Autodesk Fusion 360 part; units mm, degrees
sketch "Sketch1" plane through (0, 0, 0) normal (0, 0, 1) x (1, 0, 0)
  line L0 (30, -70) -> (-30, -70)
  line L1 (-30, -70) -> (-30, 70)
  line L2 (-30, 70) -> (30, 70)
  line L3 (30, 70) -> (30, -70)
  line L4 (30, -70) -> (-30, 70) construction
  line L5 (-30, -70) -> (30, 70) construction
  line L6 (-30, 70) -> (10, 70)
  line L7 (10, 70) -> (10, 55)
  line L8 (10, 55) -> (-30, 55)
  line L9 (-30, 55) -> (-30, 70)
  line L10 (-30, 50) -> (-25, 50)
  line L11 (-25, 50) -> (-25, 34)
  line L12 (-25, 34) -> (-30, 34)
  line L13 (-30, 34) -> (-30, 50)
  line L14 (0, 1.75) -> (0, 22.5)
  line L15 (30, 50) -> (25, 50)
  line L16 (25, 50) -> (25, 34)
  line L17 (25, 34) -> (30, 34)
  line L18 (-30, 34) -> (-25, 34)
  line L19 (-25, 34) -> (-25, 24)
  line L20 (-25, 24) -> (-30, 24)
  line L21 (-30, 24) -> (-30, 34)
  line L22 (25, 34) -> (25, 24)
  line L23 (25, 24) -> (30, 24)
  line L24 (25, 34) -> (30, 34)
  dimension "d1" = 60
  dimension "d2" = 140
  dimension "d3" = 40
  dimension "d4" = 15
  dimension "d5" = 5
  dimension "d6" = 16
  dimension "d7" = 5
  dimension "d8" = 5
  dimension "d9" = 10
extrude "Extrude1" add sketch "Sketch1" along normal blind 4 contours L0 L1 L2 L3 L7 L8 L10 L11 L15 L16 L19 L20 L22 L23
extrude "Extrude2" add sketch "Sketch1" along normal blind 12 contours L3 L17 L22 L23 L24 | L1 L12 L18 L19 L20 L21
chamfer "Chamfer1" distance 15 distance2 30 1 edges at (30, -70, 2) measured on face at (10, -70, 1.3333)
chamfer "Chamfer1" distance 30 distance2 15 1 edges at (-30, -70, 2) measured on face at (-30, 30.6667, 5.3333)
chamfer "Chamfer1" distance 1 distance2 1 4 edges at (-25, 42, 0) (-25, 42, 4) (25, 42, 4) (25, 42, 0) measured on face at (-25, 44.6667, 1.3333) measured on face at (-8.3333, -38.6667, 4) measured on face at (-8.3333, -38.6667, 4) measured on face at (-8.3333, -35.3333, 0)
chamfer "Chamfer1" distance 6 distance2 6 2 edges at (27.5, 24, 4) (-27.5, 24, 4) measured on face at (-8.3333, -38.6667, 4) measured on face at (-8.3333, -38.6667, 4)
chamfer "Chamfer1" distance 2 distance2 2 4 edges at (27.5, 24, 12) (27.5, 34, 12) (-27.5, 24, 12) (-27.5, 34, 12) measured on face at (28.3333, 30.6667, 12) measured on face at (28.3333, 30.6667, 12) measured on face at (-28.3333, 30.6667, 12) measured on face at (-28.3333, 30.6667, 12)
sketch "Sketch2" plane through (0, 0, 0) normal (1, 0, 0) x (0, 1, 0)
  circle A0 centre (29, 8) radius 1.7
  dimension "d22" = 3.4
  dimension "d23" = 29
  dimension "d24" = 8
extrude "Extrude3" cut sketch "Sketch2" along normal mid plane 100
Source: CAD feature listing. Evaluate the final solid. Frame: model axes, mm. A direction names the side the tool comes from. Round coordinates to 2 decimals unless told otherwise and drop trailing zeros. Loops run counter-clockwise (first coordinate to the right, second up) from the corner with the lowest first, then second, coordinate; pieces in that order, holes last. Notation, with made-up numbers: M -6.75,43.5 L 10.25,43.5 A21 ccw 10.25,61.5 Z; hole C 52.5,44.25 d7. An arc over 180 degrees is marked long. Use a Markdown table: item, result. Add a question column.
1. Contact query for flat-ended pins moving along their axis: P1, Ø1.8, axis at x = -27, z = 6.5, coming from the +Y side; P2, Ø1.6, axis at y = 39, z = 1.5, coming from the +X side; P3, Ø1.2, axis at x = -27, z = 3, coming from the -Y side. Output: stop coordinate, or through.
2. Line query: line 1 (Z direction, x = -28.35, y = 29); line 2 (Y direction, x = -2, z = 3); line 3 (Z direction, x = 8, y = -32.5). Output: solid intervals per line, ascending.
3. Section query A-A on z = 8. Return the cut outline in (x, y).
4. Section query B-B on y = 29. Return the cut outline in (x, z).
5. Mould query, pull axis X, two halves, no side actions, for faces 1 (the flat face through (30, 6, 3)), 2 (the flat face through (-28, 34, 5)), 3 (the flat face through (-30, 5, 3)), 4 (the flat face through (25, 28, 6)). Classes: pulls with the +X half, pulls with the -X half, needs draft (parallel to the pull), parting line crosses it, or undercut.
6. Section query D-D on x = 12.5. Return the cut outline in (y, z).
7. Reachability of faces 5 (the flat face through (-25, 28, 6)), 6 (the flat face through (22.6, -54.8, 2)), 7 (the flat face through (-10, 55, 2)) from +Z, -Z, +X, -X, +Y, -Y: full face, straight path, thin tool, end or side. Return the list, or none.
8. Section query C-C on y = 48. Return the cut outline in (x, z), then the cut area to 3 significant figures.
Reported:
| question | item | result |
|---|---|---|
| 1 | P1 | stops at y = 34 |
| 1 | P2 | stops at x = 25 |
| 1 | P3 | stops at y = -47.2 |
| 2 | line 1 | z = 0 to 6.3, 9.7 to 12 |
| 2 | line 2 | y = -70 to 55 |
| 2 | line 3 | z = 0 to 4 |
| 3 | outline | M -30,22 L -25,22 L -25,27.3 L -30,27.3 Z; M -30,30.7 L -25,30.7 L -25,34 L -30,34 Z; M 25,22 L 30,22 L 30,27.3 L 25,27.3 Z; M 25,30.7 L 30,30.7 L 30,34 L 25,34 Z |
| 4 | outline | M -30,0 L 30,0 L 30,6.3 L 25,6.3 L 25,4 L -25,4 L -25,6.3 L -30,6.3 Z; M -30,9.7 L -25,9.7 L -25,12 L -30,12 Z; M 25,9.7 L 30,9.7 L 30,12 L 25,12 Z |
| 5 | face 1 | pulls with the +X half |
| 5 | face 2 | needs draft |
| 5 | face 3 | pulls with the -X half |
| 5 | face 4 | undercut |
| 6 | outline | M -70,0 L 70,0 L 70,4 L -70,4 Z |
| 7 | face 5 | +Z, +Y, -Y |
| 7 | face 6 | +Z, -Z, +X, -Y |
| 7 | face 7 | +Z, -Z, -X, +Y |
| 8 | outline | M -25,1 L -24,0 L 24,0 L 25,1 L 25,3 L 24,4 L -24,4 L -25,3 Z |
| 8 | area | 198 mm² |
